Design review of the part built by this model. Coordinates are the model's own, in mm. A direction names the side the tool comes from. Round coordinates to 2 decimals unless told otherwise and drop trailing zeros. Write each loop counter-clockwise with the first axis right and the second up, starting at its lowest first coordinate (ties: lowest second). Pieces come first, ordered by that corner, then holes. Notation, with made-up numbers: (26, 80.25) - (54, 80.25) arc R30 ccw to (54, 111.25) - close; hole circle Ø7 at (13, -3). An arc over 180 degrees is marked (long way). Use one line per item in the form item = value.
Autodesk Inventor part; units mm, degrees
ref_plane "YZ Plane" through (0, 0, 0) normal (1, 0, 0) x (0, 1, 0)
ref_plane "XZ Plane" through (0, 0, 0) normal (0, 1, 0) x (-1, 0, 0)
ref_plane "XY Plane" through (0, 0, 0) normal (0, 0, 1) x (1, 0, 0)
sketch "Sketch1" plane through (0, 0, 0) normal (0, 0, 1) x (1, 0, 0)
  circle A0 centre (0, 0) radius 20
  circle A1 centre (0, 0) radius 6
  line L0 (0, 0) -> (-12.5, 0)
  line L1 (0, 0) -> (11.5, 0)
  circle A2 centre (-12.5, 0) radius 2.75
  circle A3 centre (11.5, 0) radius 2.75
  line L2 (0, 0) -> (-36, 0)
  circle A4 centre (-36, 0) radius 5.25
  circle A5 centre (-36, 0) radius 11
  line L3 (-36, 11) -> (0, 20)
  line L4 (-36, -11) -> (0, -20)
  line L5 (20, 0) -> (-20, 0)
  line L6 (-20, 0) -> (-20, 20)
  line L7 (-20, 20) -> (20, 20)
  line L8 (20, 20) -> (20, 0)
  line L9 (-20, 0) -> (20, 0)
  line L10 (20, 0) -> (20, -35)
  line L11 (20, -35) -> (-20, -35)
  line L12 (-20, -35) -> (-20, 0)
  point P0 (-9.4118, -17.6471)
  point P1 (-9.4118, 17.6471)
  point P2 (-20, -15)
  dimension "d0" = 40
  dimension "d1" = 12
  dimension "d2" = 12.5
  dimension "d3" = 11.5
  dimension "d4" = 5.5
  dimension "d5" = 5.5
  dimension "d8" = 36
  dimension "d9" = 10.5
  dimension "d10" = 22
  dimension "d11" = 40
  dimension "d12" = 20
  dimension "d13" = 40
  dimension "d14" = 35
extrude "Extrusion1" add sketch "Sketch1" along normal blind 10 contours L5 A3 L1 A1 L0 A2 L2 A0 L3 | L10 L11 L12 L4 A0 | A0 L4 L2 A2 L0 A1 L1 A3 L5 | L3 A0 | A0 L4 | A0 L6 L3 | L4 L12 A0 | L12 L4 A5 L2 | L2 A5 L3 L6 | A5
sketch "Sketch3" plane through (0, 0, 0) normal (0, 0, -1) x (-1, 0, 0)
  line L0 (-20, -35) -> (-20, 0)
  line L1 (-20, -35) -> (20, -35)
  line L2 (20, -35) -> (20, -6)
  line L3 (20, -6) -> (-20, -6)
  line L4 (-20, -6) -> (-20, -35)
  point P0 (0, 0)
  point P1 (-20, -6)
  dimension "d15" = 40
  dimension "d16" = 29
extrude "Extrusion2" add sketch "Sketch3" along normal blind 10
fillet "Fillet3" radius 10 1 edges at (-20, -6, -5)
fillet "Fillet4" radius 10 1 edges at (20, -6, -5)
sketch "Sketch4" plane through (20, -35, 10) normal (1, 0, 0) x (0, 0, -1)
  line L0 (20, 0) -> (0, 0)
  line L1 (0, 0) -> (20, 0)
  line L2 (20, 0) -> (20, 14)
  line L3 (20, 14) -> (0, 14)
  line L4 (0, 14) -> (0, 0)
  point P0 (10, 35)
  dimension "d23" = 20
  dimension "d24" = 14
extrude "Extrusion3" add sketch "Sketch4" along normal blind 15
sketch "Sketch5" plane through (-20, -35, -10) normal (-1, 0, 0) x (0, 0, 1)
  line L0 (0, 0) -> (0, 14)
  line L1 (20, 14) -> (20, 0)
  line L2 (0, 0) -> (20, 0)
  line L3 (20, 0) -> (20, 14)
  line L4 (20, 14) -> (0, 14)
  line L5 (0, 14) -> (0, 0)
  point P0 (10, 35)
  dimension "d27" = 20
extrude "Extrusion4" add sketch "Sketch5" along normal blind 15
sketch "Sketch6" plane through (-20, -21, 10) normal (0, 1, 0) x (1, 0, 0)
  circle A0 centre (-7.5, 15) radius 3.5
  point P0 (20, 10)
  dimension "d30" = 7
sketch "Sketch7" plane through (20, -21, 10) normal (0, 1, 0) x (1, 0, 0)
  circle A0 centre (7.273, 15) radius 3.5
  point P0 (-20, 10)
  dimension "d31" = 7
extrude "Extrusion5" cut sketch "Sketch7" against normal blind 15
extrude "Extrusion6" cut sketch "Sketch6" against normal blind 15
fillet "Fillet5" radius 5 1 edges at (35, -35, 0)
fillet "Fillet6" radius 5 1 edges at (35, -21, 0)
fillet "Fillet7" radius 5 1 edges at (-35, -35, 0)
fillet "Fillet8" radius 5 1 edges at (-35, -21, 0)
properties part number "suportCaptor"
Q1. We need section B-B on x = 11.5. Write out the cut boundary in (y, z).
Calculated:
outline = (-35, -10) - (-6.11, -10) - (-6.11, 0) - (-2.75, 0) - (-2.75, 10) - (-35, 10) - close; (2.75, 0) - (16.36, 0) - (16.36, 10) - (2.75, 10) - close
Q2. We need section D-D on y = -27.5. Write out the cut boundary in (x, z), then the cut area to 3 significant figures.
Calculated:
outline = (-35, -10) - (35, -10) - (35, 10) - (-35, 10) - close; hole circle Ø7 at (-27.5, -5); hole circle Ø7 at (27.27, -5)
area = 1,320 mm2
Q3. Machinability: for faces 1 (the flat face through (-25, -21, 0)), 2 (the flat face through (25, -21, 0)), 3 (the cylindrical face through (16.99, -8.85, -5.07)), which of the approach directions +Z, -Z, +X, -X, +Y, -Y give a long, thin tool a straight path to every point of the face, cutting with its end or side? Answer none if there is none.
Calculated:
face_1 = +Z, -Z, -X
face_2 = +Z, -Z, +X, +Y
face_3 = -Z, +X, +Y
Q4. For P1, Ø5.5, axis at x = -27.5, z = -5, coming from the -Y side; P2, Ø3, axis at x = -18, z = 3.5, coming from the +Y side (3 decimals); P3, Ø4, axis at y = -4, z = 4.5, coming from the -X side; P4, Ø3, axis at x = 24, z = -2.5, coming from the +Y side, all flat-tipped, find the tip position at first contact; note any pin that passes through.
Calculated:
P1 = through
P2 = 15.875
P3 = -46.82
P4 = -21
Q5. We need section A-A on z = 7.5. Write out the cut boundary in (x, y).
Calculated:
outline = (-36, -11) - (-19.95, -15.01) arc R10 ccw to (-20, -16) - (-20, -21) - (-30, -21) arc R5 ccw to (-35, -26) - (-35, -30) arc R5 ccw to (-30, -35) - (30, -35) arc R5 ccw to (35, -30) - (35, -26) arc R5 ccw to (30, -21) - (20, -21) - (20, 0) arc R20 ccw to (-9.41, 17.65) - (-36, 11) arc R11 ccw to start; hole circle Ø10.5 at (-36, 0); hole circle Ø5.5 at (-12.5, 0); hole circle Ø12 at (0, 0); hole circle Ø5.5 at (11.5, 0)
Q6. To check wall thickness, follow line 1 along X through (y, z) = (-26.5, -5); line 2 along Y through (x, z) = (-36, 2.75); line 3 along X through (y, z) = (-25, -5). State the ranges of each line that lie inside material, in increasing order. Write a range as from..to.
Calculated:
line_1 = -35..-31, -24..23.77, 30.77..35
line_2 = -11..-5.25, 5.25..11
line_3 = -34.92..-31, -24..23.77, 30.77..34.91
Q7. We need section C-C on y = 1. Write out the cut boundary in (x, z).
Calculated:
outline = (-46.95, 0) - (-41.15, 0) - (-41.15, 10) - (-46.95, 10) - close; (-30.85, 0) - (-15.06, 0) - (-15.06, 10) - (-30.85, 10) - close; (-9.94, 0) - (-5.92, 0) - (-5.92, 10) - (-9.94, 10) - close; (5.92, 0) - (8.94, 0) - (8.94, 10) - (5.92, 10) - close; (14.06, 0) - (19.97, 0) - (19.97, 10) - (14.06, 10) - close
Q8. Draft analysis for pull direction X (two halves, no side actions). For faces 4 (the flat face through (-28, -13, 5)), 5 (the cylindrical face through (28.9, -27.9, -1.9)), 6 (the cylindrical face through (-6, 0, 5)), 7 (the flat face through (0, -6, -5)), state which applies: released by +X, released by -X, zero draft, split by the parting line, or undercut.
Calculated:
face_4 = released by -X
face_5 = undercut
face_6 = undercut
face_7 = zero draft
